For this review, take the finished solid that the model builds, in its own axes (mm). A direction names the side the tool comes from. Coordinates: 2 decimals unless noted, no trailing zeros. Order: outer loops, then holes, each group sorted by start corner. A loop starts at its lowest first (then second) coordinate and runs counter-clockwise, first axis right, second up.
from build123d import *

# Parameters (mm, degrees)
F1_DEPTH = 8.5
F3_D     = 4.1
F3_DEPTH = 12
F3_TIP   = 1.231764269
F4_D     = 8
F4_DEPTH = 0.5
F4_TIP   = 2.4034424761


with BuildPart() as f1:
    # F0 (on Top) → F1 (new body)
    with BuildSketch(Plane.XY):
        Polygon((-21.8481650084, 5.5145221063), (-21.8481650084, 0.5145221063), (41.2518349916, 0.5145221063), (41.2518349916, 5.5145221063), (41.2518349916, 12.1145221063), (26.2518349916, 12.1145221063), (26.2518349916, 5.5145221063), (-6.8481650084, 5.5145221063), (-6.8481650084, 12.1145221063), (-21.8481650084, 12.1145221063), align=None)
    extrude(amount=F1_DEPTH)

    # F3
    with Locations(Plane.XZ.offset(-0.5145221063)):
        with Locations((-14.3481650084, 4.25), (33.7518349916, 4.25)):
            Hole(F3_D / 2, depth=F3_DEPTH)
            with Locations((0, 0, -(F3_DEPTH + F3_TIP / 2))):  # 118° drill point
                Cone(0, F3_D / 2, F3_TIP, mode=Mode.SUBTRACT)

    # F4
    with Locations(Plane.XZ.offset(-0.5145221063)):
        with Locations((-14.3481650084, 4.25), (33.7518349916, 4.25)):
            Hole(F4_D / 2, depth=F4_DEPTH)
            with Locations((0, 0, -(F4_DEPTH + F4_TIP / 2))):  # 118° drill point
                Cone(0, F4_D / 2, F4_TIP, mode=Mode.SUBTRACT)


solid = f1.part
1. Take a section at C-C, the plane y = 4.25. Give the boundary of the cut face in (x, z).
Answer below:
outline: (-21.85, 0) - (41.25, 0) - (41.25, 8.5) - (-21.85, 8.5) - close; hole circle Ø4.1 at (-14.35, 4.25); hole circle Ø4.1 at (33.75, 4.25)
2. Take a section at A-A, the plane y = 8. Give the boundary of the cut face in (x, z), plus the area to 3 significant figures.
Answer below:
outline: (-21.85, 0) - (-6.85, 0) - (-6.85, 8.5) - (-21.85, 8.5) - close; (26.25, 0) - (41.25, 0) - (41.25, 8.5) - (26.25, 8.5) - close; hole circle Ø4.1 at (-14.35, 4.25); hole circle Ø4.1 at (33.75, 4.25)
area: 229 mm2
3. Take a section at B-B, the plane z = 4.25. Give the boundary of the cut face in (x, y), plus the area to 3 significant figures.
Answer below:
outline: (-21.85, 0.51) - (-18.35, 0.51) - (-18.35, 1.01) - (-16.4, 2.19) - (-16.4, 12.11) - (-21.85, 12.11) - close; (-12.3, 2.19) - (-10.35, 1.01) - (-10.35, 0.51) - (29.75, 0.51) - (29.75, 1.01) - (31.7, 2.19) - (31.7, 12.11) - (26.25, 12.11) - (26.25, 5.51) - (-6.85, 5.51) - (-6.85, 12.11) - (-12.3, 12.11) - close; (35.8, 2.19) - (37.75, 1.01) - (37.75, 0.51) - (41.25, 0.51) - (41.25, 12.11) - (35.8, 12.11) - close
area: 410 mm2
4. Take a section at D-D, the plane x = 25. Give the boundary of the cut face in (y, z), plus the area to 3 significant figures.
Answer below:
outline: (0.51, 0) - (5.51, 0) - (5.51, 8.5) - (0.51, 8.5) - close
area: 42.5 mm2
5. Machinability: for faces 1 (the face through (10, 5.515, 4)), 2 (the face through (31.86, 7.22, 3.46)), 3 (the face through (-18.043, 0.768, 2.718)), which of the approach directions +Z, -Z, +X, -X, +Y, -Y give a long, thin tool a straight path to every point of the face, cutting with its end or side? Answer none if there is none.
Answer below:
face 1: +Z, -Z, +Y
face 2: +Y, -Y
face 3: -Y
6. The part is to be moulded in two halves that separate along X. For faces 4 (the face through (-6.848, 9, 4)), 5 (the face through (41.252, 6, 4)), 6 (the face through (36, 12.115, 2)), say which applies: +X half, -X half, draft (parallel to the pull), parting line (faces both ways), or undercut.
Answer below:
face 4: undercut
face 5: +X half
face 6: draft
7. To check wall thickness, follow L1, parallel to X at y = 0.7, z = 4.25; L2, parallel to X at y = 5, z = 4.25; L3, parallel to X at y = 10, z = 4.25. State the ranges of each line that lie inside material, in increasing order.
Answer below:
L1: x = -21.85 to -18.35, -10.35 to 29.75, 37.75 to 41.25
L2: x = -21.85 to -16.4, -12.3 to 31.7, 35.8 to 41.25
L3: x = -21.85 to -16.4, -12.3 to -6.85, 26.25 to 31.7, 35.8 to 41.25
